Read the model definition and answer for the solid it produces. Units are mm, in the model's axes. Give positions to 0.01 mm unless a question says otherwise; leave off trailing zeros. Order: outer loops, then holes, each group sorted by start corner. A loop starts at its lowest first (then second) coordinate and runs counter-clockwise, first axis right, second up. Notation, with made-up numbers: (76, 1) -> (116, 1) arc R17 cw to (116, 12) -> close; hole circle Ø11 at (87, 47). An arc over 180 degrees is marked (long way). Use one line per item in the form item = value.
```python
from build123d import *

# Parameters (mm, degrees)
F1_R     = 23.3578357485
F2_DEPTH = 1270
F3_R     = 35.7346583213
F4_DEPTH = 25.4


with BuildPart() as f2:
    # F1 (on face) → F2 (new body, symmetric)
    with BuildSketch(Plane.XZ):
        Polygon((81.899409343, 8.6979254562), (44.2631345498, 69.4546044391), (-26.7041833628, 77.9105496637), (-77.5627065371, 27.6982619059), (-70.0149296982, -43.3713820086), (-9.7444827522, -81.7814906557), (57.8637584574, -58.6084688007), align=None)
        Circle(F1_R, mode=Mode.SUBTRACT)
    extrude(amount=F2_DEPTH, both=True)

    # F3 (on face) → F4 (join)
    with BuildSketch(Plane(origin=(-73.7888181177, 0, -7.8365600513), x_dir=(0, -1, 0), z_dir=(-0.9944077718, 0, -0.1056086331))):
        with Locations((153.2169878483, 0)):
            Circle(F3_R)
    extrude(amount=F4_DEPTH)


solid = f2.part
```
Item 1: The part is cut by section A-A on y = -307.5. Give the vertices of the cut face in (x, z), and give its area (3 significant figures).
Checks:
outline = (-77.56, 27.7) -> (-70.01, -43.37) -> (-9.74, -81.78) -> (57.86, -58.61) -> (81.9, 8.7) -> (44.26, 69.45) -> (-26.7, 77.91) -> close; hole circle Ø46.72 at (0, 0)
area = 16,800 mm²
Item 2: Determine the mould class of faces 1 (the flat face through (63.345, -17.78, 38.651)), 2 (the cylindrical face through (-86.407, -117.517, -7.597)), 3 (the flat face through (-99.1, -152.7, -10)), 4 (the flat face through (-17, 1270, 17)) for opening direction X: +X half, -X half, draft (parallel to the pull), parting line (faces both ways), or undercut.
Checks:
face_1 = +X half
face_2 = undercut
face_3 = -X half
face_4 = draft
Item 3: Straight lines are drawn through the part: L1, parallel to X at y = -793, z = 9; L2, parallel to X at y = 646, z = -1.5; L3, parallel to Z at x = 0, y = -537. For each, find the intervals that lie inside material, in ascending order. Write a range as from..to.
Checks:
L1 = -75.58..-21.55, 21.55..81.71
L2 = -74.46..-23.31, 23.31..78.26
L3 = -78.44..-23.36, 23.36..74.73
Item 4: Given pin 1 Ø4 at (y, z) = (-919.5, 30.5) entering from -X; pin 2 Ø8 at (x, y) = (-72.5, -326.5) entering from -Z; pin 3 Ø4 at (y, z) = (656.5, 25.5) entering from +X, each flat-ended and moving along its own axis, determine where each tip first touches the part or whether it passes through.
Checks:
pin_1 = -76.75
pin_2 = -44.34
pin_3 = 72.73
